Could you check a few things on this model? Use its own coordinates, in mm. Face numbers are marked on the shaded views. A direction names the side the tool comes from. Give positions to 0.01 mm unless a question says otherwise; leave off trailing zeros. Loops run counter-clockwise (first coordinate to the right, second up) from the corner with the lowest first, then second, coordinate; pieces in that order, holes last. Notation, with made-up numbers: (-11, 10.5) - (17, 10.5) arc R36 cw to (17, 45.5) - close; hole circle Ø5 at (26.5, 58.25). An arc over 180 degrees is marked (long way). Answer in a Markdown table with one row per item. Add a question column.
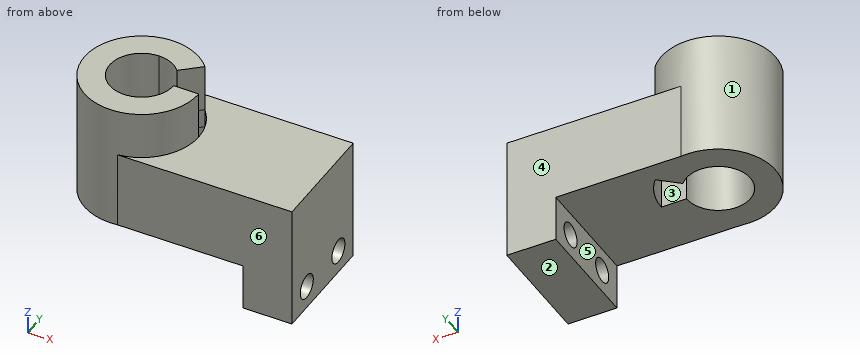
```python
from build123d import *

# Parameters (mm, degrees)
F1_DEPTH = 78.74
F2_DEPTH = 25.4
F3_DEPTH = 168.148
F4_W     = 152.277097106
F4_H     = 166.5787487769
F4_R     = 16.2034810418
F5_DEPTH = 65.786


with BuildPart() as f1:
    # F0 (on Top) → F1 (new body)
    with BuildSketch(Plane.XY):
        with BuildLine():
            Line((-76.6547471285, 42.8859197003), (-76.6547471285, 76.138548553))
            Line((-76.6547471285, 76.138548553), (-67.7737741201, 76.138548553))
            ThreePointArc((-67.7737741201, 76.138548553), (-153.309494257, 0), (-67.7737741201, -76.138548553))
            Line((-67.7737741201, -76.138548553), (-76.6547471285, -76.138548553))
            Line((-76.6547471285, -76.138548553), (-76.6547471285, -42.8859197003))
            ThreePointArc((-76.6547471285, -42.8859197003), (-119.5406668288, 0), (-76.6547471285, 42.8859197003))
        make_face()
        with BuildLine():
            Line((-67.7737741201, 76.138548553), (-76.6547471285, 76.138548553))
            Line((-76.6547471285, 76.138548553), (-76.6547471285, 42.8859197003))
            ThreePointArc((-76.6547471285, 42.8859197003), (-58.9040631626, 39.0399196629), (-44.3371342228, 28.1917364598))
            Line((-44.3371342228, 28.1917364598), (-18.8899035063, 50.3902083608))
            ThreePointArc((-18.8899035063, 50.3902083608), (-40.9313587918, 67.8217500739), (-67.7737741201, 76.138548553))
        make_face()
        with BuildLine():
            Line((100.6577461958, 76.138548553), (-67.7737741201, 76.138548553))
            ThreePointArc((-67.7737741201, 76.138548553), (-40.9313587918, 67.8217500739), (-18.8899035063, 50.3902083608))
            ThreePointArc((-18.8899035063, 50.3902083608), (-4.8776625607, 26.9072553093), (0, 0))
            ThreePointArc((0, 0), (-19.3977868636, -50.9665651046), (-67.7737741201, -76.138548553))
            Line((-67.7737741201, -76.138548553), (100.6577461958, -76.138548553))
            Line((100.6577461958, -76.138548553), (100.6577461958, 76.138548553))
        make_face()
        with BuildLine():
            Line((-76.6547471285, -76.138548553), (-67.7737741201, -76.138548553))
            ThreePointArc((-67.7737741201, -76.138548553), (-19.3977868636, -50.9665651046), (0, 0))
            Line((0, 0), (-33.7688274282, 0))
            ThreePointArc((-33.7688274282, 0), (-46.329822491, -30.3249246375), (-76.6547471285, -42.8859197003))
            Line((-76.6547471285, -42.8859197003), (-76.6547471285, -76.138548553))
        make_face()
    extrude(amount=F1_DEPTH)

    # F0 (on Top) + F1_face (on face) + F1_face1 (on face) → F2 (join)
    with BuildSketch(Plane.XY):
        with BuildLine():
            Line((-76.6547471285, 42.8859197003), (-76.6547471285, 76.138548553))
            Line((-76.6547471285, 76.138548553), (-67.7737741201, 76.138548553))
            ThreePointArc((-67.7737741201, 76.138548553), (-153.309494257, 0), (-67.7737741201, -76.138548553))
            Line((-67.7737741201, -76.138548553), (-76.6547471285, -76.138548553))
            Line((-76.6547471285, -76.138548553), (-76.6547471285, -42.8859197003))
            ThreePointArc((-76.6547471285, -42.8859197003), (-119.5406668288, 0), (-76.6547471285, 42.8859197003))
        make_face()
    with BuildSketch(Plane(origin=(-7.2978192901, -1.0520080629, 78.74), x_dir=(1, 0, 0), z_dir=(0, 0, 1))):
        with BuildLine():
            ThreePointArc((-60.47595483, 77.1905566159), (-146.0116749669, 1.0520080629), (-60.47595483, -75.08654049))
            Line((-60.47595483, -75.08654049), (107.9555654859, -75.08654049))
            Line((107.9555654859, -75.08654049), (107.9555654859, 77.1905566159))
            Line((107.9555654859, 77.1905566159), (-60.47595483, 77.1905566159))
        make_face()
        with BuildLine():
            ThreePointArc((-11.5920842162, 51.4422164237), (2.4201567294, 27.9592633723), (7.2978192901, 1.0520080629))
            Line((7.2978192901, 1.0520080629), (-26.4710081381, 1.0520080629))
            ThreePointArc((-26.4710081381, 1.0520080629), (-109.5139487719, -14.0017548647), (-37.0393149327, 29.2437445228))
            Line((-37.0393149327, 29.2437445228), (-11.5920842162, 51.4422164237))
        make_face(mode=Mode.SUBTRACT)
    with BuildSketch(Plane(origin=(-7.2978192901, -1.0520080629, 0), x_dir=(1, 0, 0), z_dir=(0, 0, -1))):
        with BuildLine():
            ThreePointArc((-60.47595483, 75.08654049), (-146.0116749669, -1.0520080629), (-60.47595483, -77.1905566159))
            Line((-60.47595483, -77.1905566159), (107.9555654859, -77.1905566159))
            Line((107.9555654859, -77.1905566159), (107.9555654859, 75.08654049))
            Line((107.9555654859, 75.08654049), (-60.47595483, 75.08654049))
        make_face()
        with BuildLine():
            ThreePointArc((7.2978192901, -1.0520080629), (2.4201567294, -27.9592633723), (-11.5920842162, -51.4422164237))
            Line((-11.5920842162, -51.4422164237), (-37.0393149327, -29.2437445228))
            ThreePointArc((-37.0393149327, -29.2437445228), (-109.5139487719, 14.0017548647), (-26.4710081381, -1.0520080629))
            Line((-26.4710081381, -1.0520080629), (7.2978192901, -1.0520080629))
        make_face(mode=Mode.SUBTRACT)
    extrude(amount=F2_DEPTH, dir=(0, 0, 1))

    # F0 (on Top) → F3 (join)
    with BuildSketch(Plane.XY):
        with BuildLine():
            Line((-76.6547471285, -76.138548553), (-67.7737741201, -76.138548553))
            ThreePointArc((-67.7737741201, -76.138548553), (-19.3977868636, -50.9665651046), (0, 0))
            Line((0, 0), (-33.7688274282, 0))
            ThreePointArc((-33.7688274282, 0), (-46.329822491, -30.3249246375), (-76.6547471285, -42.8859197003))
            Line((-76.6547471285, -42.8859197003), (-76.6547471285, -76.138548553))
        make_face()
        with BuildLine():
            Line((-76.6547471285, 42.8859197003), (-76.6547471285, 76.138548553))
            Line((-76.6547471285, 76.138548553), (-67.7737741201, 76.138548553))
            ThreePointArc((-67.7737741201, 76.138548553), (-153.309494257, 0), (-67.7737741201, -76.138548553))
            Line((-67.7737741201, -76.138548553), (-76.6547471285, -76.138548553))
            Line((-76.6547471285, -76.138548553), (-76.6547471285, -42.8859197003))
            ThreePointArc((-76.6547471285, -42.8859197003), (-119.5406668288, 0), (-76.6547471285, 42.8859197003))
        make_face()
        with BuildLine():
            Line((-67.7737741201, 76.138548553), (-76.6547471285, 76.138548553))
            Line((-76.6547471285, 76.138548553), (-76.6547471285, 42.8859197003))
            ThreePointArc((-76.6547471285, 42.8859197003), (-58.9040631626, 39.0399196629), (-44.3371342228, 28.1917364598))
            Line((-44.3371342228, 28.1917364598), (-18.8899035063, 50.3902083608))
            ThreePointArc((-18.8899035063, 50.3902083608), (-40.9313587918, 67.8217500739), (-67.7737741201, 76.138548553))
        make_face()
    extrude(amount=F3_DEPTH)

    # F4 (on face) → F5 (join)
    with BuildSketch(Plane.YZ.offset(100.6577461958)):
        with Locations((0, 20.8506256115)):
            Rectangle(F4_W, F4_H)
        with Locations((-39.326235652, -31.2090925872)):
            Circle(F4_R, mode=Mode.SUBTRACT)
        with Locations((39.326235652, -31.2090925872)):
            Circle(F4_R, mode=Mode.SUBTRACT)
    extrude(amount=F5_DEPTH)


solid = f1.part
```
(1) We'd pull the mould along X, two halves only. Please class the marked faces 1, 2 and 3: pulls with the +X half, pulls with the -X half, needs draft (parallel to the pull), parting line crosses it, or undercut.
(2) On a 3-axis mill with a long thin cutter (end or side, diameter ignored), from which of +Z, -Z, +X, -X, +Y, -Y can I reach the whole of each face in a straight line? I mean the marked faces 4, 5 and 6. Say none if no direction works.
(3) I want a section at C-C on z = -27. Please give me the cut outline in (x, y).
(4) I want a section at B-B on y = 11.5. Please give me the cut outline in (x, z).
(5) For pin 1 Ø1.5 at (x, z) = (-18.5, 28.5) entering from +Y; pin 2 Ø1.5 at (x, y) = (62.5, -37) entering from -Z; pin 3 Ø4 at (x, y) = (-54, -33) entering from -Z; pin 4 Ø1 at (x, z) = (22.5, 31.5) entering from -Y, each with a flat end and sliding along its axis, tell me the tip position at first contact or that it passes through.
(6) I want a section at D-D on z = 129.5. Please give me the cut outline in (x, y), then the cut area to 3 significant figures.
(7) Please list where these lines run through material, in increasing order: line 1 (X direction, y = 7.5, z = -46.5); line 2 (Z direction, x = 25, y = 65); line 3 (Z direction, x = 129, y = 57.5).
(8) I want a section at A-A on z = 45.5. Please give me the cut outline in (x, y), then the cut area to 3 significant figures.
Reported:
| question | item | result |
|---|---|---|
| 1 | face 1 | parting line crosses it |
| 1 | face 2 | needs draft |
| 1 | face 3 | undercut |
| 2 | face 4 | +Z, -Z, +X, +Y |
| 2 | face 5 | -Z, -X, +Y, -Y |
| 2 | face 6 | +Z, -Z, +X, -Y |
| 3 | outline | (100.66, -76.14) - (166.44, -76.14) - (166.44, -54.97) - (100.66, -54.97) - close; (100.66, -23.68) - (166.44, -23.68) - (166.44, 23.68) - (100.66, 23.68) - close; (100.66, 54.97) - (166.44, 54.97) - (166.44, 76.14) - (100.66, 76.14) - close |
| 4 | outline | (-152.44, 0) - (-117.97, 0) - (-117.97, 168.15) - (-152.44, 168.15) - close; (-0.87, 0) - (100.66, 0) - (100.66, -62.44) - (166.44, -62.44) - (166.44, 104.14) - (-0.87, 104.14) - close |
| 5 | pin 1 | y = 76.14 |
| 5 | pin 2 | z = 0 |
| 5 | pin 3 | through |
| 5 | pin 4 | y = -76.14 |
| 6 | outline | (-44.34, 28.19) - (-18.89, 50.39) arc R76.65 ccw (long way) to (0, 0) - (-33.77, 0) arc R42.89 cw (long way) to start |
| 6 | area | 11,200 mm² |
| 7 | line 1 | 100.66 to 166.44 |
| 7 | line 2 | 0 to 104.14 |
| 7 | line 3 | -62.44 to 104.14 |
| 8 | outline | (-67.77, -76.14) - (166.44, -76.14) - (166.44, 76.14) - (-67.77, 76.14) arc R76.65 ccw (long way) to start; hole (-44.34, 28.19) arc R42.89 ccw (long way) to (-33.77, 0) - (0, 0) arc R76.65 ccw to (-18.89, 50.39) - close |
| 8 | area | 39,000 mm² |
